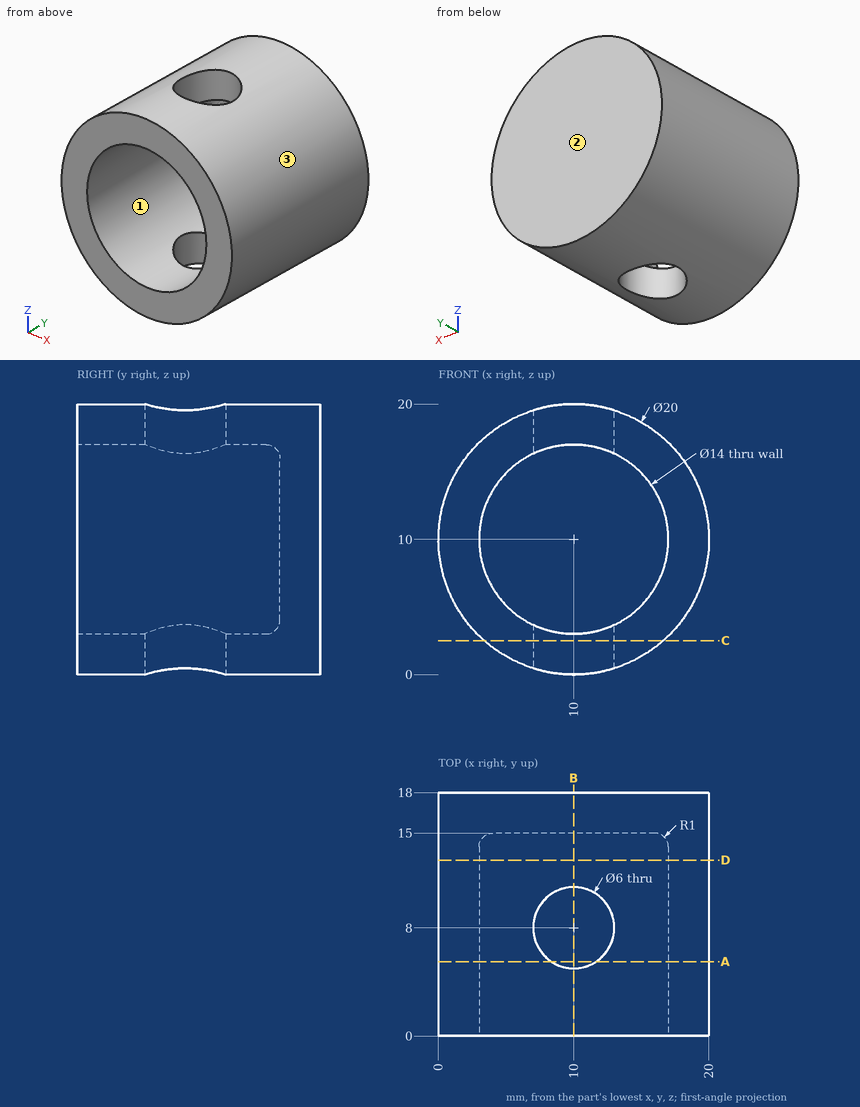
Drawing for the job (mm, zero at the part's lowest x, y, z). Round coordinates to 2 decimals unless told otherwise and drop trailing zeros. Loops run counter-clockwise (first coordinate to the right, second up) from the corner with the lowest first, then second, coordinate; pieces in that order, holes last. Notation, with made-up numbers: (31.25, 73) -> (40.25, 73) arc R19 ccw to (40.25, 81) -> close; hole circle Ø7 at (70.5, -32.75). An arc over 180 degrees is marked (long way). Answer in a Markdown table with one row per item.
Item 1: Drill centre lines: L1, parallel to X at y = 6, z = 10; L2, parallel to Y at x = 14.5, z = 8; L3, parallel to Z at x = 14.75, y = 11.5. Where is each one in solid material? Low to high. Write a range as [from, to].
Answers below:
| item | result |
|---|---|
| L1 | x = [0, 3], [17, 20] |
| L2 | y = [15, 18] |
| L3 | z = [1.2, 4.86], [15.14, 18.8] |
Item 2: Mould opens along X. For the marked faces 1, 2 and 3 say: +X half, -X half, draft (parallel to the pull), parting line (faces both ways), or undercut.
Answers below:
| item | result |
|---|---|
| face 1 | undercut |
| face 2 | draft |
| face 3 | parting line |
Item 3: Saw through at B-B (x = 10). State how many separate pieces and enclosed holes the cut face has, and give its area (3 significant figures).
Answers below:
| item | result |
|---|---|
| separate pieces | 3 |
| enclosed holes | 0 |
| area | 114 mm² |
Item 4: Saw through at C-C (z = 2.5). Write the cut outline in (x, y).
Answers below:
| item | result |
|---|---|
| outline | (3.39, 0) -> (16.61, 0) -> (16.61, 18) -> (3.39, 18) -> close; hole circle Ø6 at (10, 8) |
Item 5: Pin check, flat tips, straight feed: pin 1 (10 mm diameter, centred on y = 3, z = 17, fed in from -X); pin 2 (8 mm diameter, centred on y = 3.5, z = 4.5, fed in from +X); pin 3 (6 mm diameter, centred on x = 18, y = 10, fed in from -Z). Stop position of each tip, or through.
Answers below:
| item | result |
|---|---|
| pin 1 | stops at x = 0.2 |
| pin 2 | stops at x = 19.89 |
| pin 3 | stops at z = 1.34 |
Item 6: Saw through at A-A (y = 5.5). Write the cut outline in (x, z), and give its area (3 significant figures).
Answers below:
| item | result |
|---|---|
| outline | (8.34, 0.14) -> (8.34, 3.2) arc R7 cw to (8.34, 16.8) -> (8.34, 19.86) arc R10 ccw to start; (11.66, 0.14) arc R10 ccw to (11.66, 19.86) -> (11.66, 16.8) arc R7 cw to (11.66, 3.2) -> close |
| area | 140 mm² |
Item 7: Saw through at D-D (y = 13). Write the cut outline in (x, z).
Answers below:
| item | result |
|---|---|
| outline | circle Ø20 at (10, 10); hole circle Ø14 at (10, 10) |
